from build123d import *

# Parameters (mm, degrees)
SKETCH_1_R      = 1.6
EXTRUDE_1_DEPTH = 3
EXTRUDE_2_DEPTH = 20
FILLET_1_R      = 3


with BuildPart() as part:
    # 草图1 → 凸台-拉伸1 (new body)
    with BuildSketch(Plane.XY):
        with BuildLine():
            ThreePointArc((80.75, -26.541241493), (0, -85), (-80.75, -26.541241493))
            Line((-80.75, -26.541241493), (-95, -31.224989992))
            ThreePointArc((-95, -31.224989992), (0, -100), (95, -31.224989992))
            Line((95, -31.224989992), (80.75, -26.541241493))
        make_face()
        with Locations((-47.5, -82.27241336)):
            Circle(SKETCH_1_R, mode=Mode.SUBTRACT)
        with Locations((-82.27241336, -47.5)):
            Circle(SKETCH_1_R, mode=Mode.SUBTRACT)
        with Locations((0, -95)):
            Circle(SKETCH_1_R, mode=Mode.SUBTRACT)
        with Locations((47.5, -82.27241336)):
            Circle(SKETCH_1_R, mode=Mode.SUBTRACT)
        with Locations((82.27241336, -47.5)):
            Circle(SKETCH_1_R, mode=Mode.SUBTRACT)
    extrude(amount=EXTRUDE_1_DEPTH)

    # 草图2 → 凸台-拉伸2 (add)
    with BuildSketch(Plane.XY.offset(3)):
        with BuildLine():
            ThreePointArc((80.75, -26.541241493), (0, -85), (-80.75, -26.541241493))
            Line((-80.75, -26.541241493), (-85.975, -28.258615943))
            ThreePointArc((-85.975, -28.258615943), (0, -90.5), (85.975, -28.258615943))
            Line((85.975, -28.258615943), (80.75, -26.541241493))
        make_face()
    extrude(amount=EXTRUDE_2_DEPTH)

    # 圆角1
    fillet_1_edges = [part.edges().sort_by_distance(p)[0] for p in [
        (80.75, -26.541241493, 11.5),
        (95, -31.224989992, 1.5),
        (-95, -31.224989992, 1.5),
        (-80.75, -26.541241493, 11.5),
    ]]
    fillet(fillet_1_edges, radius=FILLET_1_R)


solid = part.part
Can you work these out from the model? Positions are in its coordinate system, mm. A direction names the side the tool comes from. Round coordinates to 2 decimals unless told otherwise and drop trailing zeros. Write each loop counter-clockwise with the first axis right and the second up, starting at its lowest first coordinate (ties: lowest second). Pieces come first, ordered by that corner, then holes. Notation, with made-up numbers: (-6.75, 42.25) - (6.25, 42.25) arc R8 cw to (6.25, 53.25) - close; hole circle Ø3 at (-15.5, 88.25). An arc over 180 degrees is marked (long way). Write each question's results on one line, items separated by ' | '. Start each with the question number.
1) Suppose I cut it at B-B (y = -66). List the corners of the cut face in (x, z) for me, and give its area (3 significant figures).
2) We'd pull the mould along Y, two halves only. Please class faces 3 (the cylindrical face through (-0.208, -93.414, 1.479)), 4 (the cylindrical face through (-1.711, -99.985, 1.479)), 5 (the flat face through (0, -91, 3)): released by +Y, released by -Y, zero draft, split by the parting line, or undercut.
3) Suppose I cut it at D-D (y = -52.5). List the corners of the cut face in (x, z) for me.
4) For pin 1 Ø8 at (y, z) = (-63.5, 7.5) entering from +X; pin 2 Ø10 at (x, z) = (-73.5, 7) entering from +Y; pin 3 Ø5 at (x, z) = (-24.5, 12.5) entering from +Y, each with a flat end and sliding along its axis, tell me the tip position at first contact or that it passes through.
5) Which directions (+Z, -Z, +X, -X, +Y, -Y) give clear straight access to the entire face, cutting with the end or side of a thin tool? Please do faces 1 (the cylindrical face through (1.451, -84.988, 11.339)), 2 (the cylindrical face through (-1.588, -90.486, 12.86)).
6) Suppose I cut it at C-C (x = -26.5). List the corners of the cut face in (y, z) for me.
7) Suppose I cut it at A-A (z = 14.5). List the corners of the cut face in (x, y) for me (3 decimals), and give its area (3 significant figures).
8) Please list where these lines run through material, in increasing order: line 1 (Z direction, x = 85, y = -42.5); line 2 (X direction, y = -71, z = 16); line 3 (Y direction, x = 47.5, z = 1).
Here are the results:
1) outline: (-75.13, 0) - (-53.56, 0) - (-53.56, 23) - (-61.92, 23) - (-61.92, 3) - (-75.13, 3) - close; (53.56, 0) - (75.13, 0) - (75.13, 3) - (61.92, 3) - (61.92, 23) - (53.56, 23) - close | area: 464 mm2
2) face 3: undercut | face 4: released by -Y | face 5: zero draft
3) outline: (-85.11, 0) - (-66.85, 0) - (-66.85, 23) - (-73.72, 23) - (-73.72, 3) - (-85.11, 3) - close; (66.85, 0) - (85.11, 0) - (85.11, 3) - (73.72, 3) - (73.72, 23) - (66.85, 23) - close
4) pin 1: stops at x = 68.19 | pin 2: stops at y = -32.6 | pin 3: stops at y = -80.6
5) face 1: +Z, -Z, +Y | face 2: +Z, -Y
6) outline: (-96.42, 0) - (-80.76, 0) - (-80.76, 23) - (-86.53, 23) - (-86.53, 3) - (-96.42, 3) - close
7) outline: (-85.975, -28.259) arc R90.5 ccw to (85.975, -28.259) - (83.551, -27.462) arc R3 ccw to (79.798, -29.279) arc R85 cw to (-79.798, -29.279) arc R3 ccw to (-83.551, -27.462) - close | area: 1,210 mm2
8) line 1: z = 0 to 3 | line 2: x = -56.12 to -46.73, 46.73 to 56.12 | line 3: y = -88 to -83.87, -80.67 to -70.49
